Answer from the drawing. Dimensions are ordinates in mm from the lowest x, y and z of the part. Coordinates: 2 decimals unless noted, no trailing zeros. Write each loop counter-clockwise with the first axis right and the second up, starting at its lowest first coordinate (ties: lowest second). Pieces come first, ordered by that corner, then holes. Notation, with made-up numbers: (-27, 80) -> (21, 80) arc R21 ccw to (21, 109) -> close; hole circle Ø9 at (-9.75, 14). An arc over 180 degrees is marked (long way). Answer as a JSON object with one key per item and string values. Group by question number.
(1) For a pull along Z with two mould halves and no side action, classify the marked faces 1, 2, 3 and 4 as +Z half, -Z half, draft (parallel to the pull), parting line (faces both ways), or undercut.
(2) Find section D-D (z = 2.5). Give the vertices of the cut face in (x, y).
(3) Find section C-C (x = 20). Give the vertices of the cut face in (y, z).
(4) Find section A-A (z = 14). Give the vertices of the cut face in (x, y) (3 decimals), then the cut area to 3 significant figures.
(5) Flat-ended cylindrical pins translate along their axes: P1, Ø5, axis at y = 27.5, z = 3, coming from the +X side; P2, Ø4, axis at x = 18, z = 11, coming from the -Y side; P3, Ø7, axis at y = 19, z = 12.5, coming from the +X side. Find the tip coordinate at first contact, or state that the pin passes through.
(6) Straight lines are drawn through the part: L1, parallel to Z at x = 15.4, y = 20 (3 decimals); L2, parallel to Z at x = 21, y = 29; L3, parallel to Z at x = 26, y = 36. For each, find the intervals that lie inside material, in ascending order.
(7) Find section B-B (y = 20). Give the vertices of the cut face in (x, z) (3 decimals), then the cut area to 3 significant figures.
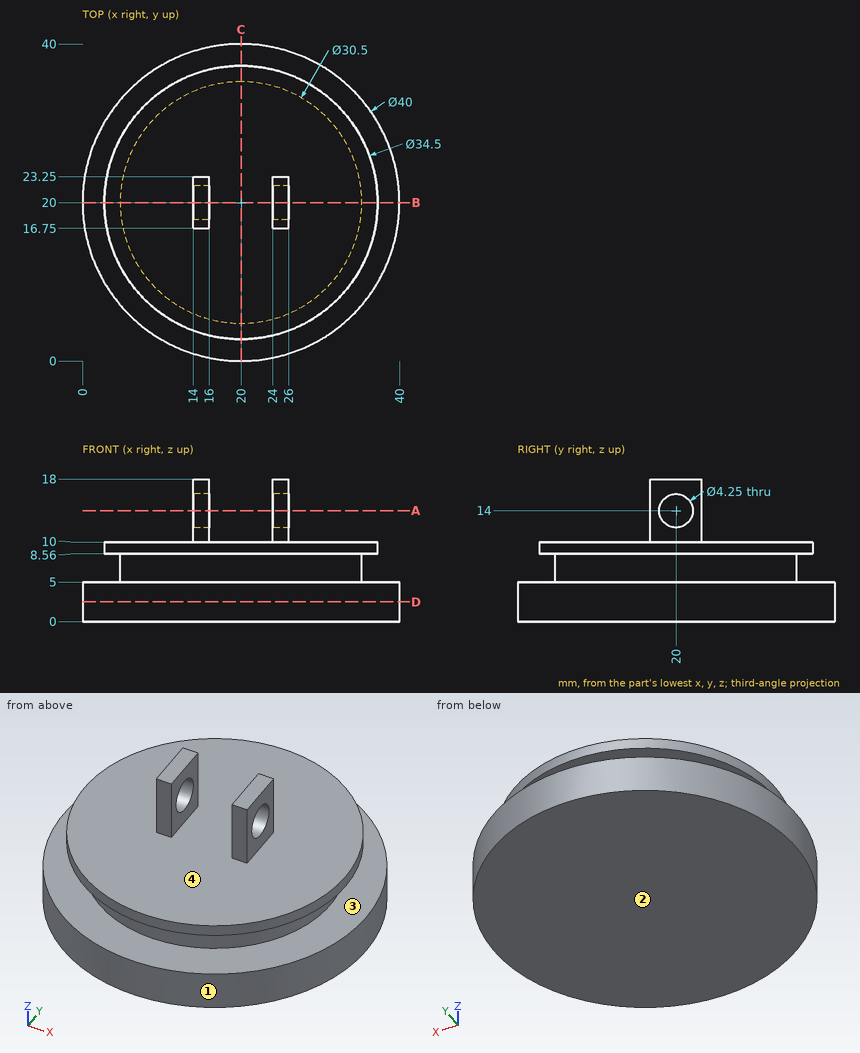
Results below:
{
 "1": {"face 1": "draft", "face 2": "-Z half", "face 3": "undercut", "face 4": "+Z half"},
 "2": {"outline": "circle Ø40 at (20, 20)"},
 "3": {"outline": "(0, 0) -> (40, 0) -> (40, 5) -> (35.25, 5) -> (35.25, 8.56) -> (37.25, 8.56) -> (37.25, 10) -> (2.75, 10) -> (2.75, 8.56) -> (4.75, 8.56) -> (4.75, 5) -> (0, 5) -> close"},
 "4": {"outline": "(14, 16.75) -> (16, 16.75) -> (16, 17.875) -> (14, 17.875) -> close; (14, 22.125) -> (16, 22.125) -> (16, 23.25) -> (14, 23.25) -> close; (24, 16.75) -> (26, 16.75) -> (26, 17.875) -> (24, 17.875) -> close; (24, 22.125) -> (26, 22.125) -> (26, 23.25) -> (24, 23.25) -> close", "area": "9.00 mm2"},
 "5": {"P1": "stops at x = 39.36", "P2": "stops at y = 2.75", "P3": "stops at x = 37.25"},
 "6": {"L1": "z = 0 to 11.875, 16.125 to 18", "L2": "z = 0 to 10", "L3": "z = 0 to 5, 8.56 to 10"},
 "7": {"outline": "(0, 0) -> (40, 0) -> (40, 5) -> (35.25, 5) -> (35.25, 8.56) -> (37.25, 8.56) -> (37.25, 10) -> (26, 10) -> (26, 11.875) -> (24, 11.875) -> (24, 10) -> (16, 10) -> (16, 11.875) -> (14, 11.875) -> (14, 10) -> (2.75, 10) -> (2.75, 8.56) -> (4.75, 8.56) -> (4.75, 5) -> (0, 5) -> close; (14, 16.125) -> (16, 16.125) -> (16, 18) -> (14, 18) -> close; (24, 16.125) -> (26, 16.125) -> (26, 18) -> (24, 18) -> close", "area": "373 mm2"}
}
